The model under review builds one solid part; all positions refer to its coordinate system, in mm. Face numbers are marked on the shaded views. Round coordinates to 2 decimals unless told otherwise and drop trailing zeros. Write each loop counter-clockwise with the first axis right and the second up, starting at its lowest first coordinate (ties: lowest second). Pieces come first, ordered by that corner, then holes. Notation, with made-up numbers: (30.5, 83) -> (88.5, 83) arc R27 cw to (88.5, 114) -> close; hole circle Ø9 at (23, -39.5). An arc over 180 degrees is marked (long way). Answer in a Markdown table with one row per item. Add a question column.
```python
from build123d import *

# Parameters (mm, degrees)
SKETCH1_W           = 23.2
SKETCH1_H           = 22.7
SKETCH1_R           = 1.6
BOSS_EXTRUDE1_DEPTH = 2
FILLET1_R           = 3
SKETCH2_R           = 0.633596253
SKETCH2_R_2         = 0.690319611
CUT_EXTRUDE1_DEPTH  = 3
SKETCH3_R           = 0.746836088
CUT_EXTRUDE2_DEPTH  = 3


with BuildPart() as part:
    # Sketch1 → Boss-Extrude1 (new body)
    with BuildSketch(Plane.XY):
        with Locations((-0.002931945, -0.247067135)):
            Rectangle(SKETCH1_W, SKETCH1_H)
        with Locations((-8.029814258, 8.024213837)):
            Circle(SKETCH1_R, mode=Mode.SUBTRACT)
        with Locations((8.021282811, 8.026881394)):
            Circle(SKETCH1_R, mode=Mode.SUBTRACT)
        with Locations((8.023950367, -8.024215675)):
            Circle(SKETCH1_R, mode=Mode.SUBTRACT)
        with Locations((-8.027146702, -8.026883232)):
            Circle(SKETCH1_R, mode=Mode.SUBTRACT)
    extrude(amount=BOSS_EXTRUDE1_DEPTH)

    # Fillet1
    fillet1_edges = [part.edges().sort_by_distance(p)[0] for p in [
        (11.597068055, -11.597067135, 1),
        (-11.602931945, -11.597067135, 1),
        (-11.602931945, 11.102932865, 1),
        (11.597068055, 11.102932865, 1),
    ]]
    fillet(fillet1_edges, radius=FILLET1_R)

    # Sketch2 → Cut-Extrude1 (cut, through all)
    with BuildSketch(Plane.XY.offset(2)):
        with Locations((6.647068055, -2.697067135)):
            Circle(SKETCH2_R)
        with Locations((6.647068055, -0.157067135)):
            Circle(SKETCH2_R)
        with Locations((6.647068055, 2.382932865)):
            Circle(SKETCH2_R)
        with Locations((-6.602931945, -4.497067135)):
            Circle(SKETCH2_R_2)
        with Locations((-6.602931945, -1.957067135)):
            Circle(SKETCH2_R_2)
        with Locations((-6.602931945, 0.582932865)):
            Circle(SKETCH2_R_2)
        with Locations((-6.602931945, 3.122932865)):
            Circle(SKETCH2_R_2)
    extrude(amount=-CUT_EXTRUDE1_DEPTH, mode=Mode.SUBTRACT)

    # Sketch3 → Cut-Extrude2 (cut, through all)
    with BuildSketch(Plane.XY.offset(2)):
        Circle(SKETCH3_R)
    extrude(amount=-CUT_EXTRUDE2_DEPTH, mode=Mode.SUBTRACT)


solid = part.part
```
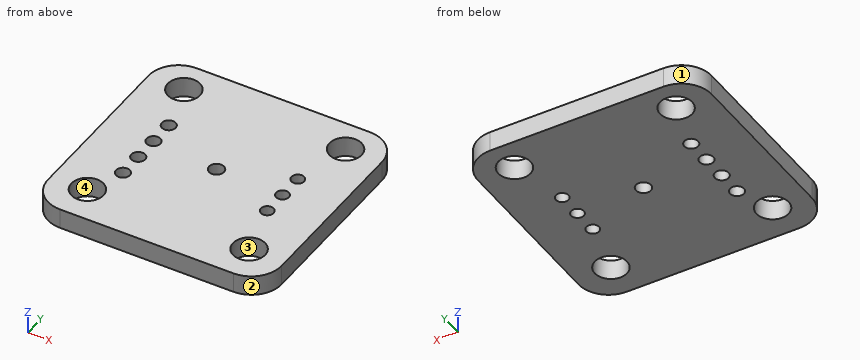
1. Insertion check: pin 1 Ø1.1 at (x, y) = (-6.6, -4.5) entering from +Z. The pin has a flat end and moves straight along its axis. Give the tip position at first contact, or say it passes through.
2. Add section C-C on z = 1.55. State how many separate pieces and enclosed holes the cut face has, plus the area to 3 significant figures.
3. Add section B-B on y = 3.5. Write out the cut boundary in (x, z).
4. For L1, parallel to Y at x = -8, z = 0.25; L2, parallel to Y at x = 7.75, z = 0.95; L3, parallel to X at y = 6.75, z = 0.35, list the stretches that pass through material, from the lowest coordinate up.
5. Add section D-D on x = -8.25. Write out the cut boundary in (y, z).
6. Mouldability with a two-part tool opening along X and no side actions: class the marked faces 1, 2, 3 and 4 as pulls with the +X half, pulls with the -X half, needs draft (parallel to the pull), parting line crosses it, or undercut.
7. Add section A-A on x = 0. Write out the cut boundary in (y, z), plus the area to 3 significant figures.
Filled in:
| question | item | result |
|---|---|---|
| 1 | pin 1 | through |
| 2 | separate pieces | 1 |
| 2 | enclosed holes | 12 |
| 2 | area | 475 mm² |
| 3 | outline | (-11.6, 0) -> (-7.18, 0) -> (-7.18, 2) -> (-11.6, 2) -> close; (-6.02, 0) -> (11.6, 0) -> (11.6, 2) -> (-6.02, 2) -> close |
| 4 | L1 | -11.6 to -9.63, -6.43 to 6.42, 9.62 to 11.1 |
| 4 | L2 | -11.6 to -9.6, -6.45 to 6.45, 9.6 to 11.1 |
| 4 | L3 | -11.6 to -9, -7.06 to 7.06, 8.99 to 11.6 |
| 5 | outline | (-11.6, 0) -> (-9.61, 0) -> (-9.61, 2) -> (-11.6, 2) -> close; (-6.44, 0) -> (6.44, 0) -> (6.44, 2) -> (-6.44, 2) -> close; (9.61, 0) -> (11.1, 0) -> (11.1, 2) -> (9.61, 2) -> close |
| 6 | face 1 | pulls with the -X half |
| 6 | face 2 | pulls with the +X half |
| 6 | face 3 | undercut |
| 6 | face 4 | undercut |
| 7 | outline | (-11.6, 0) -> (-0.75, 0) -> (-0.75, 2) -> (-11.6, 2) -> close; (0.75, 0) -> (11.1, 0) -> (11.1, 2) -> (0.75, 2) -> close |
| 7 | area | 42.4 mm² |
